```python
from build123d import *

# Parameters (mm, degrees)
BOSS_EXTRUDE1_DEPTH = 1.6
CUT_EXTRUDE2_REACH  = 74.468
SKETCH8_R           = 0.75
CUT_EXTRUDE3_REACH  = 74.468
SKETCH9_R           = 1.316483274


with BuildPart() as part:
    # Sketch1 → Boss-Extrude1 (new body)
    with BuildSketch(Plane(origin=(0, 0, 0), x_dir=(1, 0, 0), z_dir=(0, 1, 0))):
        with BuildLine():
            Line((1, 0), (64, 0))
            ThreePointArc((64, 0), (64.707106781, 0.292893219), (65, 1))
            Line((65, 1), (65, 31))
            ThreePointArc((65, 31), (64.707106781, 31.707106781), (64, 32))
            Line((64, 32), (1, 32))
            ThreePointArc((1, 32), (0.292893219, 31.707106781), (0, 31))
            Line((0, 31), (0, 1))
            ThreePointArc((0, 1), (0.292893219, 0.292893219), (1, 0))
        make_face()
    extrude(amount=BOSS_EXTRUDE1_DEPTH)

    # Sketch8 → Cut-Extrude2 (cut, up to next)
    with BuildSketch(Plane(origin=(0, 1.6, 0), x_dir=(1, 0, 0), z_dir=(0, 1, 0)), mode=Mode.PRIVATE) as cut_extrude2_sk1:
        with Locations(Location((3.5, 16, 0), (0, 0, 270))):
            Circle(SKETCH8_R)
    cut_extrude2_tool1 = extrude(cut_extrude2_sk1.sketch, amount=-CUT_EXTRUDE2_REACH, mode=Mode.PRIVATE) & part.part
    # Sketch8 → Cut-Extrude2 (cut, up to next)
    with BuildSketch(Plane(origin=(0, 1.6, 0), x_dir=(1, 0, 0), z_dir=(0, 1, 0)), mode=Mode.PRIVATE) as cut_extrude2_sk2:
        with Locations(Location((6, 18.5, 0), (0, 0, 270))):
            Circle(SKETCH8_R)
    cut_extrude2_tool2 = extrude(cut_extrude2_sk2.sketch, amount=-CUT_EXTRUDE2_REACH, mode=Mode.PRIVATE) & part.part
    # Sketch8 → Cut-Extrude2 (cut, up to next)
    with BuildSketch(Plane(origin=(0, 1.6, 0), x_dir=(1, 0, 0), z_dir=(0, 1, 0)), mode=Mode.PRIVATE) as cut_extrude2_sk3:
        with Locations(Location((6, 13.5, 0), (0, 0, 270))):
            Circle(SKETCH8_R)
    cut_extrude2_tool3 = extrude(cut_extrude2_sk3.sketch, amount=-CUT_EXTRUDE2_REACH, mode=Mode.PRIVATE) & part.part
    # Sketch8 → Cut-Extrude2 (cut, up to next)
    with BuildSketch(Plane(origin=(0, 1.6, 0), x_dir=(1, 0, 0), z_dir=(0, 1, 0)), mode=Mode.PRIVATE) as cut_extrude2_sk4:
        with Locations(Location((1, 13.499992953, 0), (0, 0, 270))):
            Circle(SKETCH8_R)
    cut_extrude2_tool4 = extrude(cut_extrude2_sk4.sketch, amount=-CUT_EXTRUDE2_REACH, mode=Mode.PRIVATE) & part.part
    # Sketch8 → Cut-Extrude2 (cut, up to next)
    with BuildSketch(Plane(origin=(0, 1.6, 0), x_dir=(1, 0, 0), z_dir=(0, 1, 0)), mode=Mode.PRIVATE) as cut_extrude2_sk5:
        with Locations(Location((1, 18.499992953, 0), (0, 0, 270))):
            Circle(SKETCH8_R)
    cut_extrude2_tool5 = extrude(cut_extrude2_sk5.sketch, amount=-CUT_EXTRUDE2_REACH, mode=Mode.PRIVATE) & part.part
    add(cut_extrude2_tool1.solids().sort_by_distance((3.5, 1.6, -16))[0], mode=Mode.SUBTRACT)
    add(cut_extrude2_tool2.solids().sort_by_distance((6, 1.6, -18.5))[0], mode=Mode.SUBTRACT)
    add(cut_extrude2_tool3.solids().sort_by_distance((6, 1.6, -13.5))[0], mode=Mode.SUBTRACT)
    add(cut_extrude2_tool4.solids().sort_by_distance((1, 1.6, -13.499993))[0], mode=Mode.SUBTRACT)
    add(cut_extrude2_tool5.solids().sort_by_distance((1, 1.6, -18.499993))[0], mode=Mode.SUBTRACT)

    # Sketch9 → Cut-Extrude3 (cut, up to next)
    with BuildSketch(Plane(origin=(0, 1.6, 0), x_dir=(1, 0, 0), z_dir=(0, 1, 0)), mode=Mode.PRIVATE) as cut_extrude3_sk1:
        with Locations(Location((43.114982321, 15.890924109, 0), (0, 0, 270))):
            Circle(SKETCH9_R)
    cut_extrude3_tool1 = extrude(cut_extrude3_sk1.sketch, amount=-CUT_EXTRUDE3_REACH, mode=Mode.PRIVATE) & part.part
    add(cut_extrude3_tool1.solids().sort_by_distance((43.114982, 1.6, -15.890924))[0], mode=Mode.SUBTRACT)


solid = part.part
```
CAD build for the part. Positions are in the model's coordinates, mm. Coordinates: 2 decimals unless noted, no trailing zeros. Write each loop counter-clockwise with the first axis right and the second up, starting at its lowest first coordinate (ties: lowest second). Pieces come first, ordered by that corner, then holes.
(1) Cut at B-B, the plane z = -18.5. List the corners of the cut face in (x, y), and give its area (3 significant figures).
(2) Two-plate mould, pull along X, no slides. Class faces 1 (the face through (65, 1, -16)), 2 (the face through (3.044, 0.811, -16.595)), 3 (the face through (0, 1, -16)): +X half, -X half, draft (parallel to the pull), parting line (faces both ways), or undercut.
(3) Drill centre lines: probe 1 along X at (y, z) = (0.6, -18.5); probe 2 along X at (y, z) = (1.15, -18); probe 3 along Z at (x, y) = (42.5, 0.4). Where is each one in solid material? Low to high.
(4) Cut at A-A, the plane x = 3.5. List the corners of the cut face in (y, z).
(5) Flat gauge pin, fed straight in: pin 1 (1.2 mm diameter, centred on x = 6, z = -13.5, fed in from -Y). Where does the tip first touch, or does it go through?
Geometry says:
1. outline: (0, 0) - (0.25, 0) - (0.25, 1.6) - (0, 1.6) - close; (1.75, 0) - (5.25, 0) - (5.25, 1.6) - (1.75, 1.6) - close; (6.75, 0) - (65, 0) - (65, 1.6) - (6.75, 1.6) - close
1. area: 99.2 mm2
2. face 1: +X half
2. face 2: undercut
2. face 3: -X half
3. probe 1: x = 0 to 0.25, 1.75 to 5.25, 6.75 to 65
3. probe 2: x = 0 to 0.44, 1.56 to 5.44, 6.56 to 65
3. probe 3: z = -32 to -17.05, -14.73 to 0
4. outline: (0, -32) - (1.6, -32) - (1.6, -16.75) - (0, -16.75) - close; (0, -15.25) - (1.6, -15.25) - (1.6, 0) - (0, 0) - close
5. pin 1: passes through
